from build123d import *

# Parameters (mm, degrees)
SKETCH1_W           = 20.32
SKETCH1_H           = 15.24
BOSS_EXTRUDE1_DEPTH = 4.9609375
CAVITY1_START       = -4.9609375
CAVITY1_OUTLINE_W   = 5.08
CAVITY1_OUTLINE_H   = 4.9609375
CAVITY1_DEPTH       = 9.921875


# Read off the part's stored shape, not the designer's step: Cavity1
with BuildPart() as part:
    # Sketch1 → Boss-Extrude1 (new body)
    with BuildSketch(Plane.XY):
        Rectangle(SKETCH1_W, SKETCH1_H)
    extrude(amount=BOSS_EXTRUDE1_DEPTH)

    # Cavity1 outline → Cavity1 (cut)
    with BuildSketch(Plane.YZ.offset(CAVITY1_START)):
        with Locations((0, 2.48046875)):
            Rectangle(CAVITY1_OUTLINE_W, CAVITY1_OUTLINE_H)
    extrude(amount=CAVITY1_DEPTH, mode=Mode.SUBTRACT)


solid = part.part
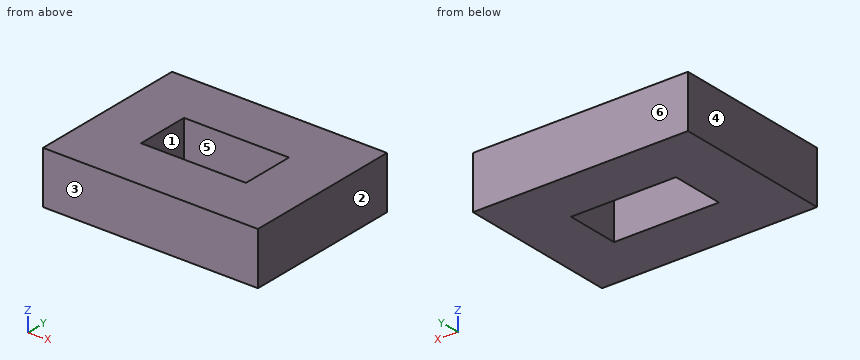
Geometry check sheet. Reference: the model listing, model coordinates, mm. Face numbers are marked on the shaded views. A direction names the side the tool comes from. Give positions to 0.01 mm unless a question says otherwise; leave off trailing zeros. Order: outer loops, then holes, each group sorted by start corner. A loop starts at its lowest first (then second) coordinate and runs counter-clockwise, first axis right, second up.
1) Cross-section at C-C (z = 2.05). Record the boundary of the cut face in (x, y), then the cut area to 3 significant figures.
Results are:
outline: (-10.16, -7.62) - (10.16, -7.62) - (10.16, 7.62) - (-10.16, 7.62) - close; hole (-4.96, -2.54) - (4.96, -2.54) - (4.96, 2.54) - (-4.96, 2.54) - close
area: 259 mm2
2) Cross-section at B-B (x = 1.75). Record the boundary of the cut face in (y, z).
Results are:
outline: (-7.62, 0) - (-2.54, 0) - (-2.54, 4.96) - (-7.62, 4.96) - close; (2.54, 0) - (7.62, 0) - (7.62, 4.96) - (2.54, 4.96) - close
3) Tool access check on the marked faces 1 and 2. Record the directions out of +Z, -Z, +X, -X, +Y, -Y that give a thin tool (end or side, any length) a straight path to the whole face; none if there is none.
Results are:
face 1: +Z, -Z
face 2: +Z, -Z, +X, +Y, -Y
4) Draft check along Y on the marked faces 3, 4, 5 and 6. Enter one of: released by +Y, released by -Y, zero draft, split by the parting line, or undercut.
Results are:
face 3: released by -Y
face 4: zero draft
face 5: undercut
face 6: released by +Y
5) Material ranges on probe 1 along Y at (x, z) = (3.25, 1.1); probe 2 along X at (y, z) = (2.5, 1), recorded low to high.
Results are:
probe 1: y = -7.62 to -2.54, 2.54 to 7.62
probe 2: x = -10.16 to -4.96, 4.96 to 10.16
6) Cross-section at A-A (y = -1.5). Record the boundary of the cut face in (x, z).
Results are:
outline: (-10.16, 0) - (-4.96, 0) - (-4.96, 4.96) - (-10.16, 4.96) - close; (4.96, 0) - (10.16, 0) - (10.16, 4.96) - (4.96, 4.96) - close
